The figure shows three views and two pictorial views of one solid part (mm, origin at its lowest corner). Answer the questions. A direction names the side the tool comes from. Give positions to 0.01 mm unless a question says otherwise; leave off trailing zeros. Order: outer loops, then holes, each group sorted by start corner. A loop starts at its lowest first (then second) coordinate and runs counter-clockwise, first axis right, second up. Notation, with made-up numbers: M -5,4 L 54,4 A12 ccw 54,25 Z; hole C 44.25,50 d3. An arc over 180 degrees is marked long. One line per item, written item: value.
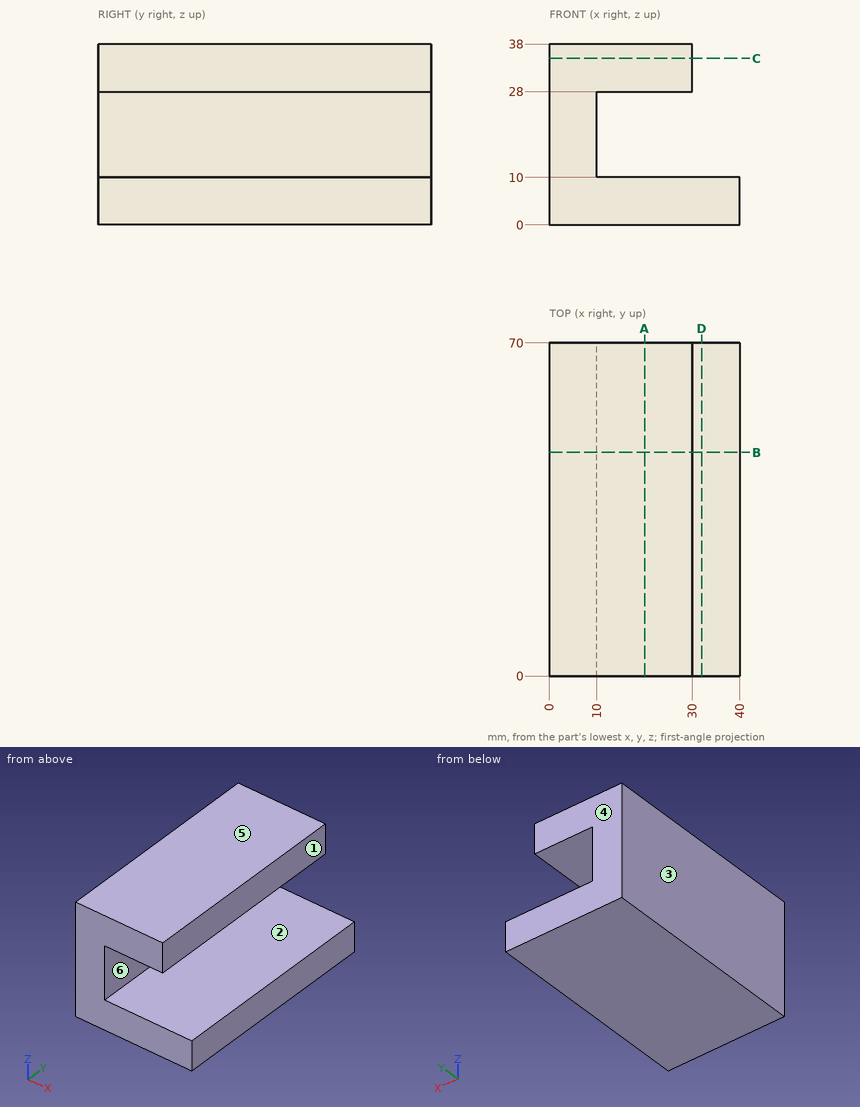
1) Determine the mould class of the marked faces 4, 5 and 6 for opening direction Z: +Z half, -Z half, draft (parallel to the pull), parting line (faces both ways), or undercut.
Reported:
face 4: draft
face 5: +Z half
face 6: undercut
2) Find section C-C, the plane z = 35. Write down the section's boundary in (x, y), plus the area to 3 significant figures.
Reported:
outline: M 0,0 L 30,0 L 30,70 L 0,70 Z
area: 2,100 mm^2
3) Find section B-B, the plane y = 47. Write down the section's boundary in (x, z).
Reported:
outline: M 0,0 L 40,0 L 40,10 L 10,10 L 10,28 L 30,28 L 30,38 L 0,38 Z
4) Find section A-A, the plane x = 20. Write down the section's boundary in (y, z).
Reported:
outline: M 0,0 L 70,0 L 70,10 L 0,10 Z; M 0,28 L 70,28 L 70,38 L 0,38 Z
5) Consider probe 1 along Z at (x, y) = (19.5, 48.5); probe 2 along X at (y, z) = (12, 24.5). Determine where each line is inside the solid, lowest interval first.
Reported:
probe 1: z = 0 to 10, 28 to 38
probe 2: x = 0 to 10
6) Which of the six approach directions +Z, -Z, +X, -X, +Y, -Y give full straight-line access (tool end or side, diameter ignored) to the marked faces 1, 2 and 3?
Reported:
face 1: +Z, +X, +Y, -Y
face 2: +X, +Y, -Y
face 3: +Z, -Z, -X, +Y, -Y
7) Find section D-D, the plane x = 32. Write down the section's boundary in (y, z), plus the area to 3 significant figures.
Reported:
outline: M 0,0 L 70,0 L 70,10 L 0,10 Z
area: 700 mm^2
8) Each of these flat-tipped pins is pushed along its axis until it touches: pin 1 Ø6 at (x, z) = (8, 31) entering from -Y; pin 2 Ø8 at (y, z) = (44, 30.5) entering from +X; pin 3 Ø5.5 at (y, z) = (42, 15.5) entering from +X; pin 4 Ø1.5 at (x, y) = (31, 10) entering from +Z. Where does it stop, or does it pass through?
Reported:
pin 1: stops at y = 0
pin 2: stops at x = 30
pin 3: stops at x = 10
pin 4: stops at z = 10
